For this review, take the finished solid that the model builds, in its own axes (mm). Face numbers are marked on the shaded views. Coordinates: 2 decimals unless noted, no trailing zeros. Loops run counter-clockwise (first coordinate to the right, second up) from the corner with the lowest first, then second, coordinate; pieces in that order, holes last. Notation, with made-up numbers: (68, 47.5) - (111, 47.5) arc R15 ccw to (111, 62.5) - close; hole circle Ø9 at (-26.75, -21.75). An arc over 180 degrees is marked (long way). One line per item, written item: value. Start each with the question number.
1. Take a section at A-A, the plane z = -4. State the section outline as (x, y) points (3 decimals).
2. Take a section at C-C, the plane y = 0.9. State the section outline as (x, z) points (3 decimals), and give its area (3 significant figures).
3. Insertion check: pin 1 (1.5 mm diameter, centred on x = 3.5, z = -5, fed in from -Y). The pin has a flat end and moves straight along its axis. Give the tip position at first contact, or say it passes through.
4. To check wall thickness, follow line 1 (Z direction, x = 2.35, y = 0.4); line 2 (Z direction, x = 3.65, y = 0.1); line 3 (X direction, y = 0.7, z = -4.75). State the ranges of each line that lie inside material, in increasing order. Write a range as from..to.
5. Take a section at B-B, the plane x = 1.45. State the section outline as (y, z) points, and give its area (3 significant figures).
6. The part is to be moulded in two halves that separate along X. For the marked faces 1, 2, 3 and 4, say which applies: released by +X, released by -X, zero draft, split by the parting line, or undercut.
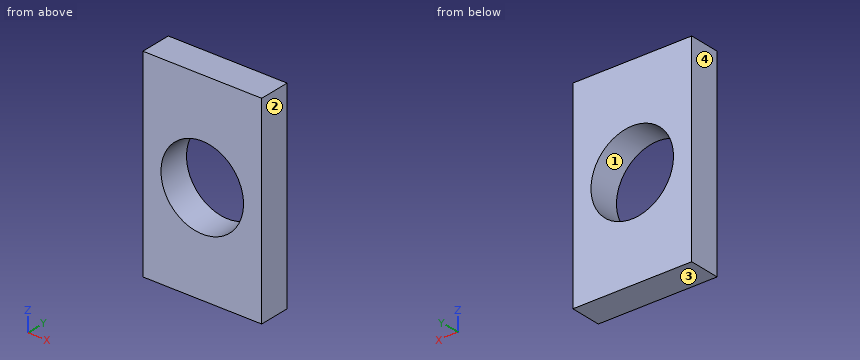
```python
from build123d import *

# Parameters (mm, degrees)
SKETCH1_W             = 4.75
SKETCH1_H             = 8
BOSS_EXTRUDE1_DEPTH   = 1.25
M4X0_7_TAPPED_HOLE1_D = 3.3


with BuildPart() as part:
    # Sketch1 → Boss-Extrude1 (new body)
    with BuildSketch(Plane(origin=(0, 0, 0), x_dir=(1, 0, 0), z_dir=(0, 1, 0))):
        with Locations((2.375, 4)):
            Rectangle(SKETCH1_W, SKETCH1_H)
    extrude(amount=BOSS_EXTRUDE1_DEPTH)

    # M4x0.7 Tapped Hole1 (through all)
    with Locations(Plane(origin=(0, 1.25, 0), x_dir=(1, 0, 0), z_dir=(0, 1, 0))):
        with Locations((2.375, 4)):
            Hole(M4X0_7_TAPPED_HOLE1_D / 2)


solid = part.part
```
Solutions:
1. outline: (0, 0) - (0.725, 0) - (0.725, 1.25) - (0, 1.25) - close; (4.025, 0) - (4.75, 0) - (4.75, 1.25) - (4.025, 1.25) - close
2. outline: (0, -8) - (4.75, -8) - (4.75, 0) - (0, 0) - close; hole circle Ø3.3 at (2.375, -4)
2. area: 29.4 mm2
3. pin 1: y = 0
4. line 1: -8..-5.65, -2.35..0
4. line 2: -8..-5.05, -2.95..0
4. line 3: 0..0.91, 3.84..4.75
5. outline: (0, -8) - (1.25, -8) - (1.25, -5.37) - (0, -5.37) - close; (0, -2.63) - (1.25, -2.63) - (1.25, 0) - (0, 0) - close
5. area: 6.58 mm2
6. face 1: undercut
6. face 2: released by +X
6. face 3: zero draft
6. face 4: released by -X
